Input: part model. Units: mm. Frame: model coordinates. A direction names the side the tool comes from. Give positions to 0.01 mm unless a question says otherwise; leave off trailing zeros. Order: outer loops, then holes, each group sorted by start corner. A loop starts at its lowest first (then second) coordinate and runs counter-clockwise, first axis right, second up. Notation, with made-up numbers: (83.25, 61) - (103.25, 61) arc R15 ccw to (103.25, 78) - close; hole circle Ø5 at (17, 81). An arc over 180 degrees is marked (long way). Use a Markdown table: item, result.
from build123d import *

# Parameters (mm, degrees)
BOSS_EXTRUDE1_DEPTH = 12.7
SKETCH2_R           = 3.175
CUT_EXTRUDE1_DEPTH  = 12.7
SKETCH3_R           = 3.175
CUT_EXTRUDE2_DEPTH  = 12.7


with BuildPart() as part:
    # Sketch1 → Boss-Extrude1 (new body)
    with BuildSketch(Plane.XY):
        Polygon((-30.762128425, 2.921), (-30.762128425, -12.954), (-14.887128425, -12.954), (-14.887128425, -9.779), (-27.587128425, -9.779), (-27.587128425, 2.921), align=None)
    extrude(amount=BOSS_EXTRUDE1_DEPTH)

    # Sketch2 → Cut-Extrude1 (cut)
    with BuildSketch(Plane(origin=(-27.587128425, 0, 0), x_dir=(0, 0, -1), z_dir=(1, 0, 0))):
        with Locations((-6.35, -3.429)):
            Circle(SKETCH2_R)
    extrude(amount=-CUT_EXTRUDE1_DEPTH, mode=Mode.SUBTRACT)

    # Sketch3 → Cut-Extrude2 (cut)
    with BuildSketch(Plane(origin=(0, -9.779, 0), x_dir=(1, 0, 0), z_dir=(0, 1, 0))):
        with Locations(Location((-21.237128425, -6.35, 0), (0, 0, 180))):
            Circle(SKETCH3_R)
    extrude(amount=-CUT_EXTRUDE2_DEPTH, mode=Mode.SUBTRACT)


solid = part.part
1. Section query A-A (z = 6.35). Return loops of the section in (x, y).
Response:
| item | result |
|---|---|
| outline | (-30.76, -12.95) - (-24.41, -12.95) - (-24.41, -9.78) - (-27.59, -9.78) - (-27.59, -6.6) - (-30.76, -6.6) - close; (-30.76, -0.25) - (-27.59, -0.25) - (-27.59, 2.92) - (-30.76, 2.92) - close; (-18.06, -12.95) - (-14.89, -12.95) - (-14.89, -9.78) - (-18.06, -9.78) - close |
2. Section query C-C (y = -12). Return loops of the section in (x, z) (3 decimals), then the cut area to 3 significant figures.
Response:
| item | result |
|---|---|
| outline | (-30.762, 0) - (-14.887, 0) - (-14.887, 12.7) - (-30.762, 12.7) - close; hole circle Ø6.35 at (-21.237, 6.35) |
| area | 170 mm^2 |
3. Set-up query: faces 4 (the face through (-30.762, -7, 6)), 5 (the face through (-27.587, -5, 3)). Return all of +Z, -Z, +X, -X, +Y, -Y with unobstructed straight access to the full face (end or side cutting, diameter ignored); none if empty.
Response:
| item | result |
|---|---|
| face 4 | +Z, -Z, -X, +Y, -Y |
| face 5 | +Z, -Z, +X, +Y |
4. Mould query, pull axis Y, two halves, no side actions, for faces 1 (the face through (-25, -12.954, 6)), 2 (the face through (-29, 2.921, 6)), 3 (the face through (-29.2, -4.6, 3.4)). Classes: pulls with the +Y half, pulls with the -Y half, needs draft (parallel to the pull), parting line crosses it, or undercut.
Response:
| item | result |
|---|---|
| face 1 | pulls with the -Y half |
| face 2 | pulls with the +Y half |
| face 3 | undercut |
5. Material intervals for line 1 along Y through (x, z) = (-29, 6.35); line 2 along Y through (x, z) = (-24.5, 9.75); line 3 along X through (y, z) = (-1.25, 12.25), sorted ascending.
Response:
| item | result |
|---|---|
| line 1 | y = -12.95 to -6.6, -0.25 to 2.92 |
| line 2 | y = -12.95 to -9.78 |
| line 3 | x = -30.76 to -27.59 |
6. Pin query (flat end, axial travel): pin 1 (3 mm diameter, centred on x = -19.5, z = 5.5, fed in from -Y); pin 2 (6 mm diameter, centred on x = -22.5, z = 9.5, fed in from +Y); pin 3 (4 mm diameter, centred on y = -5, z = 4, fed in from +X). Return the tip coordinate at first contact, or that it passes through.
Response:
| item | result |
|---|---|
| pin 1 | stops at y = -12.95 |
| pin 2 | stops at y = -9.78 |
| pin 3 | stops at x = -27.59 |
7. Section query B-B (y = -1.25). Return loops of the section in (x, z), then the cut area to 3 significant figures.
Response:
| item | result |
|---|---|
| outline | (-30.76, 0) - (-27.59, 0) - (-27.59, 4.04) - (-30.76, 4.04) - close; (-30.76, 8.66) - (-27.59, 8.66) - (-27.59, 12.7) - (-30.76, 12.7) - close |
| area | 25.7 mm^2 |
8. Section query D-D (z = 11.5). Return loops of the section in (x, y).
Response:
| item | result |
|---|---|
| outline | (-30.76, -12.95) - (-14.89, -12.95) - (-14.89, -9.78) - (-27.59, -9.78) - (-27.59, 2.92) - (-30.76, 2.92) - close |
